Source: CAD feature listing. Evaluate the final solid. Frame: model axes, mm. Coordinates: 2 decimals unless noted, no trailing zeros. Write each loop counter-clockwise with the first axis right and the second up, starting at its lowest first coordinate (ties: lowest second). Pieces come first, ordered by that corner, then holes. Notation, with made-up numbers: (-38.75, 43) - (-10.75, 43) arc R17 ccw to (-10.75, 55) - close; hole circle Ø2 at (-35.75, 70.25). An arc over 180 degrees is marked (long way). One line per item, written item: value.
from build123d import *

# Parameters (mm, degrees)
CUT_EXTRUDE_1_DEPTH = 1.2
CUT_EXTRUDE_2_DEPTH = 1.2
SKETCH_4_R          = 4
CUT_EXTRUDE_3_DEPTH = 10
CHAMFER_1_SIZE      = 0.5
FILLET_1_R          = 0.2
FILLET_2_R          = 0.2
CHAMFER_2_SIZE      = 0.5
CHAMFER_3_SIZE      = 0.5
FILLET_3_R          = 0.2


with BuildPart() as part:
    # Эскиз1 → Повернуть1 (revolve)
    with BuildSketch(Plane(origin=(0, 0, 0), x_dir=(0, 0, -1), z_dir=(1, 0, 0)), mode=Mode.PRIVATE) as revolve_1_sk:
        Polygon((0, 0), (0, 3), (35, 3), (35, 10), (51, 10), (51, 11), (1145, 11), (1145, 10), (1185, 10), (2375, 10), (2375, 3), (2410, 3), (2410, 0), align=None)
    revolve(revolve_1_sk.sketch.rotate(Axis((0, 0, 0), (0, 0, -1)), 90), axis=Axis((0, 0, 0), (0, 0, -1)))

    # Эскиз2 → Вырез-Вытянуть1 (cut)
    with BuildSketch(Plane(origin=(0, 10, 0), x_dir=(1, 0, 0), z_dir=(0, 1, 0))):
        with BuildLine():
            Line((3, 47), (3, 39))
            ThreePointArc((3, 39), (0, 36), (-3, 39))
            Line((-3, 39), (-3, 47))
            ThreePointArc((-3, 47), (0, 50), (3, 47))
        make_face()
    extrude(amount=-CUT_EXTRUDE_1_DEPTH, mode=Mode.SUBTRACT)

    # Эскиз3 → Вырез-Вытянуть2 (cut)
    with BuildSketch(Plane(origin=(0, 10, 0), x_dir=(1, 0, 0), z_dir=(0, 1, 0))):
        with BuildLine():
            Line((3, 2371), (3, 2363))
            ThreePointArc((3, 2363), (0, 2360), (-3, 2363))
            Line((-3, 2363), (-3, 2371))
            ThreePointArc((-3, 2371), (0, 2374), (3, 2371))
        make_face()
    extrude(amount=-CUT_EXTRUDE_2_DEPTH, mode=Mode.SUBTRACT)

    # Эскиз4 → Вырез-Вытянуть3 (cut)
    with BuildSketch(Plane(origin=(0, 10, 0), x_dir=(1, 0, 0), z_dir=(0, 1, 0))):
        with Locations(Location((0, 1155, 0), (0, 0, 270))):
            Circle(SKETCH_4_R)
    extrude(amount=-CUT_EXTRUDE_3_DEPTH, mode=Mode.SUBTRACT)

    # Фаска1
    chamfer_1_edges = [part.edges().sort_by_distance(p)[0] for p in [
        (-3, 0, 0),
        (-10, 0, -35),
        (-11, 0, -51),
    ]]
    chamfer(chamfer_1_edges, length=CHAMFER_1_SIZE)

    # Скругление1
    fillet_1_edges = [part.edges().sort_by_distance(p)[0] for p in [
        (-10, 0, -51),
    ]]
    fillet(fillet_1_edges, radius=FILLET_1_R)

    # Скругление2
    fillet_2_edges = [part.edges().sort_by_distance(p)[0] for p in [
        (-10, 0, -1145),
    ]]
    fillet(fillet_2_edges, radius=FILLET_2_R)

    # Фаска2
    chamfer_2_edges = [part.edges().sort_by_distance(p)[0] for p in [
        (-11, 0, -1145),
    ]]
    chamfer(chamfer_2_edges, length=CHAMFER_2_SIZE)

    # Фаска3
    chamfer_3_edges = [part.edges().sort_by_distance(p)[0] for p in [
        (-10, 0, -2375),
        (-3, 0, -2410),
    ]]
    chamfer(chamfer_3_edges, length=CHAMFER_3_SIZE)

    # Скругление3
    fillet_3_edges = [part.edges().sort_by_distance(p)[0] for p in [
        (-3, 0, -2375),
    ]]
    fillet(fillet_3_edges, radius=FILLET_3_R)


solid = part.part
1) Section query A-A on z = -940.5. Output: boundary loops of the cut face in (x, y), then the cut area to 3 significant figures.
Values found:
outline: circle Ø22 at (0, 0)
area: 380 mm2
2) Section query B-B on z = -2105. Output: boundary loops of the cut face in (x, y).
Values found:
outline: circle Ø20 at (0, 0)
3) Material intervals for line 1 (X direction, y = 3.25, z = -1155); line 2 (Z direction, x = 0, y = 3.5); line 3 (Z direction, x = 5, y = 7.5), sorted ascending.
Values found:
line 1: -9.46 to -4, 4 to 9.46
line 2: -2375 to -1159, -1151 to -35
line 3: -2375 to -35
4) Contact query for flat-ended pins moving along their axis: P1, Ø10, axis at y = -5.5, z = -614, coming from the +X side; P2, Ø4, axis at x = -1.5, z = -1157, coming from the +Y side; P3, Ø9, axis at x = 0, z = -1155, coming from the -Y side. Output: stop coordinate, or through.
Values found:
P1: x = 10.99
P2: y = 9.96
P3: y = -10
